from build123d import *

# Parameters (mm, degrees)
SKETCH1_W                                        = 101.6
SKETCH1_H                                        = 101.6
BOSS_EXTRUDE1_DEPTH                              = 10
CBORE_FOR_6_BUTTON_HEAD_CAP_SCREW1_D             = 3.7973
CBORE_FOR_6_BUTTON_HEAD_CAP_SCREW1_CBORE_D       = 7.54126
CBORE_FOR_6_BUTTON_HEAD_CAP_SCREW1_CBORE_DEPTH   = 5.08
CBORE_FOR_1_4_SOCKET_HEAD_CAP_SCREW1_D           = 6.7564
CBORE_FOR_1_4_SOCKET_HEAD_CAP_SCREW1_CBORE_D     = 11.1125
CBORE_FOR_1_4_SOCKET_HEAD_CAP_SCREW1_CBORE_DEPTH = 6.35
SKETCH8_W                                        = 76.2
SKETCH8_H                                        = 11.1125
CUT_EXTRUDE1_DEPTH                               = 6.35
SKETCH10_W                                       = 76.2
SKETCH10_H                                       = 6.7564
CUT_EXTRUDE2_DEPTH                               = 135.853429693


with BuildPart() as part:
    # Sketch1 → Boss-Extrude1 (new body)
    with BuildSketch(Plane.XY):
        with Locations((-44.45, -44.45)):
            Rectangle(SKETCH1_W, SKETCH1_H)
    extrude(amount=BOSS_EXTRUDE1_DEPTH)

    # CBORE for #6 Button Head Cap Screw1 (through all)
    with Locations(Plane.XY.offset(10)):
        with Locations((0, 0), (0, -88.9), (-88.9, -88.9), (-88.9, 0)):
            CounterBoreHole(CBORE_FOR_6_BUTTON_HEAD_CAP_SCREW1_D / 2, CBORE_FOR_6_BUTTON_HEAD_CAP_SCREW1_CBORE_D / 2, CBORE_FOR_6_BUTTON_HEAD_CAP_SCREW1_CBORE_DEPTH)

    # CBORE for 1/4 Socket Head Cap Screw1 (through all)
    with Locations(Plane(origin=(0, 0, 0), x_dir=(-1, 0, 0), z_dir=(0, 0, -1))):
        with Locations((82.55, -19.05), (82.55, -69.85), (6.35, -69.85), (6.35, -19.05)):
            CounterBoreHole(CBORE_FOR_1_4_SOCKET_HEAD_CAP_SCREW1_D / 2, CBORE_FOR_1_4_SOCKET_HEAD_CAP_SCREW1_CBORE_D / 2, CBORE_FOR_1_4_SOCKET_HEAD_CAP_SCREW1_CBORE_DEPTH)

    # Sketch8 → Cut-Extrude1 (cut)
    with BuildSketch(Plane(origin=(0, 0, 0), x_dir=(-1, 0, 0), z_dir=(0, 0, -1))):
        with Locations((44.45, -19.05)):
            Rectangle(SKETCH8_W, SKETCH8_H)
        with Locations((44.45, -69.85)):
            Rectangle(SKETCH8_W, SKETCH8_H)
    extrude(amount=-CUT_EXTRUDE1_DEPTH, mode=Mode.SUBTRACT)

    # Sketch10 → Cut-Extrude2 (cut, through all)
    with BuildSketch(Plane(origin=(0, 0, 6.35), x_dir=(-1, 0, 0), z_dir=(0, 0, -1))):
        with Locations((44.45, -19.05)):
            Rectangle(SKETCH10_W, SKETCH10_H)
        with Locations((44.45, -69.85)):
            Rectangle(SKETCH10_W, SKETCH10_H)
    extrude(amount=-CUT_EXTRUDE2_DEPTH, mode=Mode.SUBTRACT)


solid = part.part
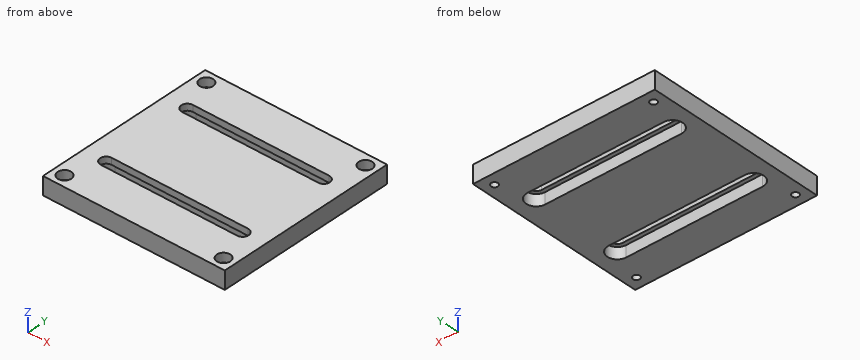
Could you check a few things on this model? Use its own coordinates, in mm. Coordinates: 2 decimals unless noted, no trailing zeros. Loops run counter-clockwise (first coordinate to the right, second up) from the corner with the lowest first, then second, coordinate; pieces in that order, holes last.
1. I need wall thicknesses on L1, parallel to Y at x = 0, z = 6.1; L2, parallel to Y at x = -44, z = 6.5; L3, parallel to X at y = -88.9, z = 3.5. Which ranges of each line are inside material? Lowest first, please.
2. Imagine slicing it at A-A (y = -88.9). Please give me the cut outline in (x, z).
3. Imagine slicing it at C-C (y = -19.05). Please give me the cut outline in (x, z), and give its area (3 significant figures).
4. For P1, Ø6, axis at x = -88.9, y = -88.9, coming from the +Z side, with a flat end and sliding along its axis, tell me the tip position at first contact or that it passes through.
5. Imagine slicing it at B-B (x = -14). Please give me the cut outline in (y, z).
6. Imagine slicing it at D-D (z = 1.5). Please give me the cut outline in (x, y).
Computed values:
1. L1: y = -95.25 to -92.67, -85.13 to -3.77, 3.77 to 6.35
1. L2: y = -95.25 to -73.23, -66.47 to -22.43, -15.67 to 6.35
1. L3: x = -95.25 to -90.8, -87 to -1.9, 1.9 to 6.35
2. outline: (-95.25, 0) - (-90.8, 0) - (-90.8, 4.92) - (-92.67, 4.92) - (-92.67, 10) - (-95.25, 10) - close; (-87, 0) - (-1.9, 0) - (-1.9, 4.92) - (-3.77, 4.92) - (-3.77, 10) - (-85.13, 10) - (-85.13, 4.92) - (-87, 4.92) - close; (1.9, 0) - (6.35, 0) - (6.35, 10) - (3.77, 10) - (3.77, 4.92) - (1.9, 4.92) - close
3. outline: (-95.25, 0) - (-88.11, 0) - (-88.11, 6.35) - (-85.93, 6.35) - (-85.93, 10) - (-95.25, 10) - close; (-2.97, 6.35) - (-0.79, 6.35) - (-0.79, 0) - (6.35, 0) - (6.35, 10) - (-2.97, 10) - close
3. area: 159 mm2
4. P1: stops at z = 4.92
5. outline: (-95.25, 0) - (-75.41, 0) - (-75.41, 6.35) - (-73.23, 6.35) - (-73.23, 10) - (-95.25, 10) - close; (-66.47, 6.35) - (-64.29, 6.35) - (-64.29, 0) - (-24.61, 0) - (-24.61, 6.35) - (-22.43, 6.35) - (-22.43, 10) - (-66.47, 10) - close; (-15.67, 6.35) - (-13.49, 6.35) - (-13.49, 0) - (6.35, 0) - (6.35, 10) - (-15.67, 10) - close
6. outline: (-95.25, -95.25) - (6.35, -95.25) - (6.35, 6.35) - (-95.25, 6.35) - close; hole circle Ø3.8 at (-88.9, -88.9); hole circle Ø3.8 at (-88.9, 0); hole (-82.55, -75.41) - (-6.35, -75.41) arc R5.56 ccw to (-6.35, -64.29) - (-82.55, -64.29) arc R5.56 ccw to start; hole (-82.55, -24.61) - (-6.35, -24.61) arc R5.56 ccw to (-6.35, -13.49) - (-82.55, -13.49) arc R5.56 ccw to start; hole circle Ø3.8 at (0, -88.9); hole circle Ø3.8 at (0, 0)
